Input: part model. Units: mm. Frame: model coordinates. Face numbers are marked on the shaded views. Round coordinates to 2 decimals unless told otherwise and drop trailing zeros. Write each loop counter-clockwise with the first axis right and the second up, starting at its lowest first coordinate (ties: lowest second). Pieces come first, ordered by that corner, then holes. Notation, with made-up numbers: (-20, 74.5) -> (13, 74.5) arc R30 ccw to (13, 110.5) -> close; hole circle Ø2 at (68.5, 50). An arc over 180 degrees is marked (long way). Write item = value, one per line.
```python
from build123d import *

# Parameters (mm, degrees)
CROQUIS2_W              = 65
CROQUIS2_H              = 55
CROQUIS2_R              = 1.5
SALIENTE_EXTRUIR1_DEPTH = 5
CROQUIS4_W              = 65
CROQUIS4_H              = 55
CROQUIS4_R              = 3.5
SALIENTE_EXTRUIR2_DEPTH = 25
CROQUIS6_R              = 12.5
CORTAR_EXTRUIR1_DEPTH   = 60
CROQUIS7_R              = 6.5
CORTAR_EXTRUIR2_DEPTH   = 5
CROQUIS8_R              = 1.5
CORTAR_EXTRUIR3_DEPTH   = 10
CROQUIS9_W              = 6
CROQUIS9_H              = 3
CORTAR_EXTRUIR6_DEPTH   = 10


with BuildPart() as part:
    # Croquis2 → Saliente-Extruir1 (new body)
    with BuildSketch(Plane(origin=(0, 0, 0), x_dir=(1, 0, 0), z_dir=(0, 1, 0))):
        with Locations((32.5, 27.5)):
            Rectangle(CROQUIS2_W, CROQUIS2_H)
        with Locations(Location((5, 50, 0), (0, 0, 270))):
            Circle(CROQUIS2_R, mode=Mode.SUBTRACT)
        with Locations(Location((32.5, 50, 0), (0, 0, 270))):
            Circle(CROQUIS2_R, mode=Mode.SUBTRACT)
        with Locations(Location((60, 50, 0), (0, 0, 270))):
            Circle(CROQUIS2_R, mode=Mode.SUBTRACT)
        with Locations(Location((5, 5, 0), (0, 0, 270))):
            Circle(CROQUIS2_R, mode=Mode.SUBTRACT)
        with Locations(Location((32.5, 5, 0), (0, 0, 270))):
            Circle(CROQUIS2_R, mode=Mode.SUBTRACT)
        with Locations(Location((60, 5, 0), (0, 0, 270))):
            Circle(CROQUIS2_R, mode=Mode.SUBTRACT)
    extrude(amount=SALIENTE_EXTRUIR1_DEPTH)

    # Croquis4 → Saliente-Extruir2 (add)
    with BuildSketch(Plane(origin=(0, 5, 0), x_dir=(1, 0, 0), z_dir=(0, 1, 0))):
        with Locations((32.5, 27.5)):
            Rectangle(CROQUIS4_W, CROQUIS4_H)
        with Locations(Location((5, 50, 0), (0, 0, 270))):
            Circle(CROQUIS4_R, mode=Mode.SUBTRACT)
        with Locations(Location((32.5, 50, 0), (0, 0, 270))):
            Circle(CROQUIS4_R, mode=Mode.SUBTRACT)
        with Locations(Location((60, 50, 0), (0, 0, 270))):
            Circle(CROQUIS4_R, mode=Mode.SUBTRACT)
        with Locations(Location((60, 5, 0), (0, 0, 270))):
            Circle(CROQUIS4_R, mode=Mode.SUBTRACT)
        with Locations(Location((32.5, 5, 0), (0, 0, 270))):
            Circle(CROQUIS4_R, mode=Mode.SUBTRACT)
        with Locations(Location((5, 5, 0), (0, 0, 270))):
            Circle(CROQUIS4_R, mode=Mode.SUBTRACT)
    extrude(amount=SALIENTE_EXTRUIR2_DEPTH)

    # Croquis6 → Cortar-Extruir1 (cut)
    with BuildSketch(Plane(origin=(65, 0, 0), x_dir=(0, 0, -1), z_dir=(1, 0, 0))):
        with Locations((27.5, 0)):
            Circle(CROQUIS6_R)
    extrude(amount=-CORTAR_EXTRUIR1_DEPTH, mode=Mode.SUBTRACT)

    # Croquis7 → Cortar-Extruir2 (cut)
    with BuildSketch(Plane.ZY):
        with Locations((-27.5, 0)):
            Circle(CROQUIS7_R)
    extrude(amount=-CORTAR_EXTRUIR2_DEPTH, mode=Mode.SUBTRACT)

    # Croquis8 → Cortar-Extruir3 (cut)
    with BuildSketch(Plane(origin=(0, 30, 0), x_dir=(1, 0, 0), z_dir=(0, 1, 0))):
        with Locations(Location((18.75, 50, 0), (0, 0, 270))):
            Circle(CROQUIS8_R)
        with Locations(Location((46.25, 50, 0), (0, 0, 270))):
            Circle(CROQUIS8_R)
        with Locations(Location((46.25, 5, 0), (0, 0, 270))):
            Circle(CROQUIS8_R)
        with Locations(Location((18.75, 5, 0), (0, 0, 270))):
            Circle(CROQUIS8_R)
    extrude(amount=-CORTAR_EXTRUIR3_DEPTH, mode=Mode.SUBTRACT)

    # Croquis9 → Cortar-Extruir6 (cut)
    with BuildSketch(Plane.XY):
        with Locations((18.75, 23.5)):
            Rectangle(CROQUIS9_W, CROQUIS9_H)
        with Locations((46.25, 23.5)):
            Rectangle(CROQUIS9_W, CROQUIS9_H)
    cortar_extruir6 = extrude(amount=-CORTAR_EXTRUIR6_DEPTH, mode=Mode.SUBTRACT)

    # Simetría1: Cortar-Extruir6 across plane
    add(cortar_extruir6.mirror(Plane.XY.offset(-27.5)), mode=Mode.SUBTRACT)


solid = part.part
```
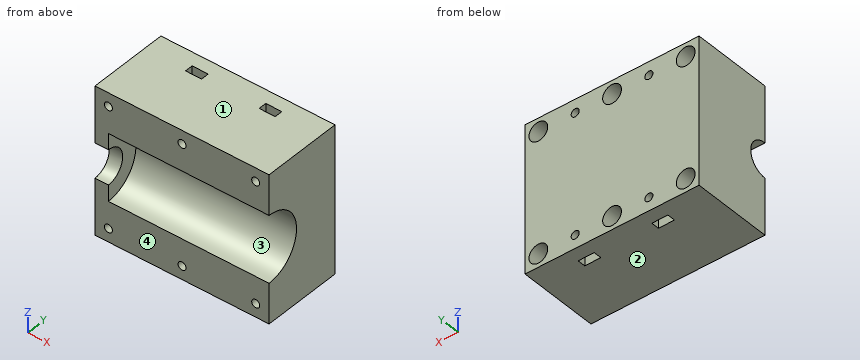
1) Line query: L1, parallel to X at y = 27.5, z = -50; L2, parallel to X at y = 3.95, z = -5; L3, parallel to X at y = 7.25, z = -53. Output: solid intervals per line, ascending. Write a range as from..to.
Solutions:
L1 = 0..1.5, 8.5..17.25, 20.25..29, 36..44.75, 47.75..56.5, 63.5..65
L2 = 0..3.5, 6.5..31, 34..58.5, 61.5..65
L3 = 0..3.2, 6.8..30.7, 34.3..58.2, 61.8..65
2) First-contact query: P1, Ø1, axis at y = 7.5, z = -32.5, coming from the +X side; P2, Ø2.5, axis at x = 60, z = -50, coming from the -Y side; P3, Ø0.9, axis at x = 46.5, z = -50.5, coming from the +Y side; P4, Ø4, axis at x = 21, z = -35, coming from the -Y side. Flat tips, straight axial feed; report the tip coordinate or a pass-through.
Solutions:
P1 = 5
P2 = through
P3 = 20
P4 = 8.12
3) Cut plane B-B (y = 15.5). Return the cut outline in (x, z).
Solutions:
outline = (0, -55) -> (65, -55) -> (65, 0) -> (0, 0) -> close; hole circle Ø7 at (5, -50); hole circle Ø7 at (5, -5); hole circle Ø7 at (32.5, -50); hole circle Ø7 at (32.5, -5); hole circle Ø7 at (60, -50); hole circle Ø7 at (60, -5)
4) Cut plane C-C (y = 2.25). Return the cut outline in (x, z), and give its area (3 significant figures).
Solutions:
outline = (0, -55) -> (65, -55) -> (65, -39.8) -> (5, -39.8) -> (5, -33.6) -> (0, -33.6) -> close; (0, -21.4) -> (5, -21.4) -> (5, -15.2) -> (65, -15.2) -> (65, 0) -> (0, 0) -> close; hole circle Ø3 at (5, -50); hole circle Ø3 at (5, -5); hole circle Ø3 at (32.5, -50); hole circle Ø3 at (32.5, -5); hole circle Ø3 at (60, -50); hole circle Ø3 at (60, -5)
area = 2,000 mm^2
5) Cut plane A-A (x = 18.75). Count the separate pieces of the cut face and the enclosed holes in it, and give its area (3 significant figures).
Solutions:
separate_pieces = 3
enclosed_holes = 0
area = 1,300 mm^2
6) Draft query along Z for the marked faces 1, 2, 3 and 4. Return one class per face: +Z half, -Z half, draft (parallel to the pull), parting line (faces both ways), or undercut.
Solutions:
face_1 = +Z half
face_2 = -Z half
face_3 = undercut
face_4 = draft
